```python
from build123d import *

# Parameters (mm, degrees)
CYLINDER_SKETCH_R              = 6.35
CYLINDER_DEPTH                 = 50.8
SKETCH2_W                      = 6.5278
SKETCH2_H                      = 49.8
SKETCH2_W_2                    = 3.81
SKETCH2_H_2                    = 1
CUT_EXTRUDE2_DEPTH             = 3.2639
CUT_EXTRUDE2_DIRECTION_2_REACH = 8.35
FILLET1_R                      = 0.3


with BuildPart() as part:
    # cylinder_sketch → cylinder (new body)
    with BuildSketch(Plane(origin=(0, 0, 0), x_dir=(1, 0, 0), z_dir=(0, 1, 0))):
        Circle(CYLINDER_SKETCH_R)
    extrude(amount=CYLINDER_DEPTH)

    # Sketch2 → Cut-Extrude2 (cut)
    with BuildSketch(Plane.XY):
        with Locations((0, 24.9)):
            Rectangle(SKETCH2_W, SKETCH2_H)
        with Locations((0, 50.3)):
            Rectangle(SKETCH2_W_2, SKETCH2_H_2)
    extrude(amount=-CUT_EXTRUDE2_DEPTH, mode=Mode.SUBTRACT)

    # Sketch2 → Cut-Extrude2 direction 2 (cut, up to next)
    with BuildSketch(Plane.XY, mode=Mode.PRIVATE) as cut_extrude2_direction_2_sk1:
        with Locations((0, 24.9)):
            Rectangle(SKETCH2_W, SKETCH2_H)
    cut_extrude2_direction_2_tool1 = extrude(cut_extrude2_direction_2_sk1.sketch, amount=CUT_EXTRUDE2_DIRECTION_2_REACH, mode=Mode.PRIVATE) & part.part
    add(cut_extrude2_direction_2_tool1.solids().sort_by_distance((0, 24.9, 0))[0], mode=Mode.SUBTRACT)
    # Sketch2 → Cut-Extrude2 direction 2 (cut, up to next)
    with BuildSketch(Plane.XY, mode=Mode.PRIVATE) as cut_extrude2_direction_2_sk2:
        with Locations((0, 50.3)):
            Rectangle(SKETCH2_W_2, SKETCH2_H_2)
    cut_extrude2_direction_2_tool2 = extrude(cut_extrude2_direction_2_sk2.sketch, amount=CUT_EXTRUDE2_DIRECTION_2_REACH, mode=Mode.PRIVATE) & part.part
    add(cut_extrude2_direction_2_tool2.solids().sort_by_distance((0, 50.3, 0))[0], mode=Mode.SUBTRACT)

    # Fillet1
    fillet1_edges = [part.edges().sort_by_distance(p)[0] for p in [
        (1.905, 49.8, 1.396806964),
        (-1.905, 49.8, 1.396806964),
        (-3.2639, 0, 1.091533835),
        (3.2639, 0, 1.091533835),
    ]]
    fillet(fillet1_edges, radius=FILLET1_R)


solid = part.part
```
Input: part model. Units: mm. Frame: model coordinates. A direction names the side the tool comes from. Give positions to 0.01 mm unless a question says otherwise; leave off trailing zeros. Loops run counter-clockwise (first coordinate to the right, second up) from the corner with the lowest first, then second, coordinate; pieces in that order, holes last.
1) Reachability of faces 1 (the flat face through (3.264, 25, 1)), 2 (the flat face through (3, 50.8, 0)) from +Z, -Z, +X, -X, +Y, -Y: full face, straight path, thin tool, end or side. Return the list, or none.
A:
face 1: +Z, -Y
face 2: +Z, -Z, +X, -X, +Y
2) Line query: L1, parallel to X at y = 20, z = -2.75; L2, parallel to X at y = 38.5, z = 0.5; L3, parallel to Y at x = 2.5, z = 2.75. Output: solid intervals per line, ascending.
A:
L1: x = -5.72 to -3.26, 3.26 to 5.72
L2: x = -6.33 to -3.26, 3.26 to 6.33
L3: y = 49.8 to 50.8
3) Contact query for flat-ended pins moving along their axis: pin 1 (1.5 mm diameter, centred on y = 42.5, z = -3.5, fed in from +X); pin 2 (3 mm diameter, centred on y = 15, z = -4, fed in from -X); pin 3 (6 mm diameter, centred on y = 23.5, z = -4.5, fed in from +X); pin 4 (1.2 mm diameter, centred on x = 3, z = 0.5, fed in from -Y). Output: stop coordinate, or through.
A:
pin 1: stops at x = 5.72
pin 2: stops at x = -5.84
pin 3: stops at x = 6.17
pin 4: stops at y = 0
4) Section query C-C on y = 45.5. Return the cut outline in (x, z), and give its area (3 significant figures).
A:
outline: (-3.26, -3.26) - (-3.26, 5.45) arc R6.35 ccw (long way) to (3.26, 5.45) - (3.26, -3.26) - close
area: 65.8 mm2
5) Section query B-B on x = 0. Return the cut outline in (y, z), and give its area (3 significant figures).
A:
outline: (0, -6.35) - (50.8, -6.35) - (50.8, -3.26) - (0, -3.26) - close
area: 157 mm2
6) Section query D-D on z = 3.5. Return the cut outline in (x, y) (3 decimals).
A:
outline: (-5.298, 0) - (-3.564, 0) arc R0.3 ccw to (-3.264, 0.3) - (-3.264, 49.8) - (-2.205, 49.8) arc R0.3 ccw to (-1.905, 50.1) - (-1.905, 50.8) - (-5.298, 50.8) - close; (1.905, 50.1) arc R0.3 ccw to (2.205, 49.8) - (3.264, 49.8) - (3.264, 0.3) arc R0.3 ccw to (3.564, 0) - (5.298, 0) - (5.298, 50.8) - (1.905, 50.8) - close
7) Section query A-A on z = 0. Return the cut outline in (x, y) (3 decimals), and give its area (3 significant figures).
A:
outline: (-6.35, 0) - (-3.564, 0) arc R0.3 ccw to (-3.264, 0.3) - (-3.264, 49.8) - (-2.205, 49.8) arc R0.3 ccw to (-1.905, 50.1) - (-1.905, 50.8) - (-6.35, 50.8) - close; (1.905, 50.1) arc R0.3 ccw to (2.205, 49.8) - (3.264, 49.8) - (3.264, 0.3) arc R0.3 ccw to (3.564, 0) - (6.35, 0) - (6.35, 50.8) - (1.905, 50.8) - close
area: 316 mm2
